Part print with two shaded views. Sizes in mm from the minimum x, y, z corner. A direction names the side the tool comes from. Coordinates: 2 decimals unless noted, no trailing zeros. Order: outer loops, then holes, each group sorted by start corner. A loop starts at its lowest first (then second) coordinate and runs counter-clockwise, first axis right, second up. Notation, with made-up numbers: (27.25, 12) - (55.25, 12) arc R17 ccw to (55.25, 19) - close; hole circle Ø3 at (58.5, 45.25). An arc over 180 degrees is marked (long way). Return JSON: item names as keys, results as strings.
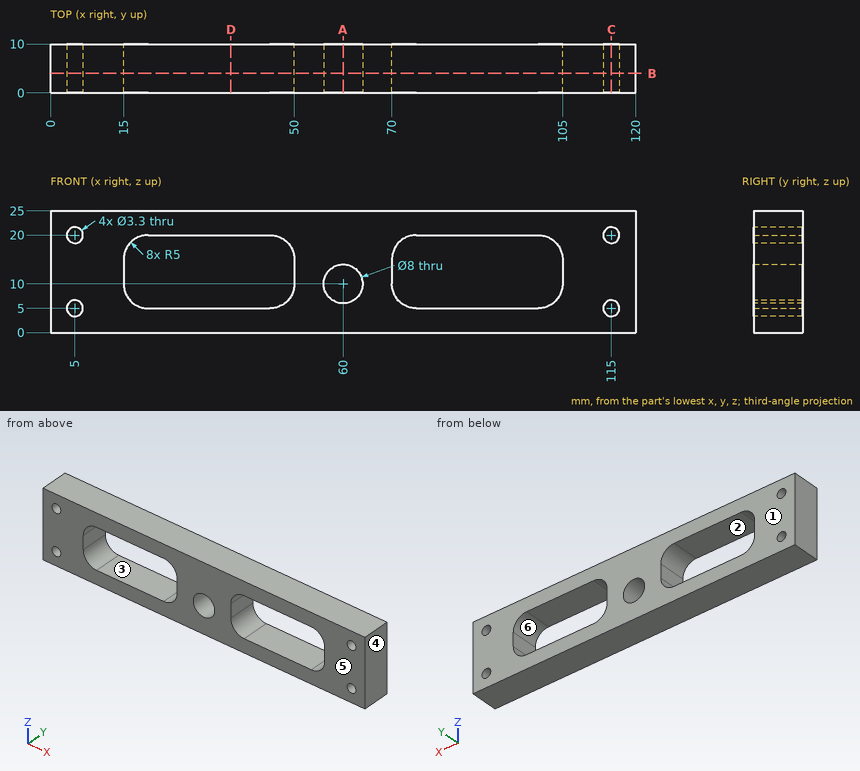
Item 1: Which spindle directions (+Z, -Z, +X, -X, +Y, -Y) get a long thin tool onto all of the face, cutting with end or side? Do the marked faces 1 and 2. Say none if no direction does.
Findings below:
{"face 1": "+Z, -Z, +X, -X, +Y", "face 2": "+Y, -Y"}
Item 2: Band-saw the part on D-D, the plane x = 37. List the corners of the cut face in (y, z).
Findings below:
{"outline": "(0, 0) - (10, 0) - (10, 5) - (0, 5) - close; (0, 20) - (10, 20) - (10, 25) - (0, 25) - close"}
Item 3: Drop a flat-ended pin along its axis: P1, Ø2, axis at x = 5, z = 20, coming from the -Y side. Give the stop position or say it passes through.
Findings below:
{"P1": "passes through"}
Item 4: Wall check: L1, parallel to X at y = 2.5, z = 14.75; L2, parallel to X at y = 2.5, z = 4.75; L3, parallel to Z at x = 5, y = 7.25. Give the ranges that are in metal, low to high. Write a range as [from, to].
Findings below:
{"L1": "x = [0, 15], [50, 70], [105, 120]", "L2": "x = [0, 3.37], [6.63, 113.37], [116.63, 120]", "L3": "z = [0, 3.35], [6.65, 18.35], [21.65, 25]"}
Item 5: Band-saw the part on C-C, the plane x = 115. List the corners of the cut face in (y, z).
Findings below:
{"outline": "(0, 0) - (10, 0) - (10, 3.35) - (0, 3.35) - close; (0, 6.65) - (10, 6.65) - (10, 18.35) - (0, 18.35) - close; (0, 21.65) - (10, 21.65) - (10, 25) - (0, 25) - close"}
Item 6: Mould opens along X. For the marked faces 3, 4, 5 and 6 say: released by +X, released by -X, zero draft, split by the parting line, or undercut.
Findings below:
{"face 3": "undercut", "face 4": "released by +X", "face 5": "zero draft", "face 6": "undercut"}
Item 7: Band-saw the part on A-A, the plane x = 60. List the corners of the cut face in (y, z).
Findings below:
{"outline": "(0, 0) - (10, 0) - (10, 6) - (0, 6) - close; (0, 14) - (10, 14) - (10, 25) - (0, 25) - close"}
Item 8: Band-saw the part on B-B, the plane y = 4. List the corners of the cut face in (x, z), then the cut area to 3 significant figures.
Findings below:
{"outline": "(0, 0) - (120, 0) - (120, 25) - (0, 25) - close; hole circle Ø3.3 at (5, 5); hole circle Ø3.3 at (5, 20); hole (15, 10) arc R5 ccw to (20, 5) - (45, 5) arc R5 ccw to (50, 10) - (50, 15) arc R5 ccw to (45, 20) - (20, 20) arc R5 ccw to (15, 15) - close; hole circle Ø8 at (60, 10); hole (70, 10) arc R5 ccw to (75, 5) - (100, 5) arc R5 ccw to (105, 10) - (105, 15) arc R5 ccw to (100, 20) - (75, 20) arc R5 ccw to (70, 15) - close; hole circle Ø3.3 at (115, 5); hole circle Ø3.3 at (115, 20)", "area": "1,910 mm²"}
